```python
from build123d import *

# Parameters (mm, degrees)
F1_DEPTH     = 25.4
F2_R         = 17.018
F3_DEPTH     = 27.686
F4_R         = 35.7378
F5_DEPTH     = 24.638
F6_R         = 17.7830971004
F7_DEPTH     = 25.4
F8_W         = 71.4756
F8_H         = 155.2468025039
F9_DEPTH     = 24.638
F10_R        = 17.78
F12_T1_DEPTH = 35.9156
F12_T3_DEPTH = 26.5465599919
F12_T6_ANGLE = 90
F12_T8_ANGLE = 90


# Not quite as in the source:
# - a fillet or chamfer that OpenCascade refuses, or shapes differently, is made with other operations: its cross-section is extruded or revolved along the edge and cut away or added


with BuildPart() as f1:
    # F0 (on Top) → F1 (new body)
    with BuildSketch(Plane.XY):
        with BuildLine():
            Line((-43.18, 0), (43.18, 0))
            ThreePointArc((43.18, 0), (0, 43.18), (-43.18, 0))
        make_face()
        with BuildLine():
            ThreePointArc((-43.18, 0), (0, -43.18), (43.18, 0))
            Line((43.18, 0), (-43.18, 0))
        make_face()
    extrude(amount=F1_DEPTH)

    # F2 (on face) → F3 (cut)
    with BuildSketch(Plane.XY):
        Circle(F2_R)
    extrude(amount=F3_DEPTH, mode=Mode.SUBTRACT)

    # F4 (on face) → F5 (cut)
    with BuildSketch(Plane.XY.offset(25.4)):
        Circle(F4_R)
    extrude(amount=-F5_DEPTH, mode=Mode.SUBTRACT)

    # F6
    f6_edges = [f1.edges().sort_by_distance(p)[0] for p in [
        (-35.7378, 0, 0.762),
    ]]
    fillet(f6_edges, radius=F6_R)

    # F0 (on Top) → F7 (join)
    with BuildSketch(Plane.XY):
        with BuildLine():
            Line((43.18, -150.0849872828), (43.18, 0))
            ThreePointArc((43.18, 0), (0, -43.18), (-43.18, 0))
            Line((-43.18, 0), (-43.18, -150.0849872828))
            Line((-43.18, -150.0849872828), (43.18, -150.0849872828))
        make_face()
    extrude(amount=F7_DEPTH)

    # F8 (on face) → F9 (cut)
    with BuildSketch(Plane.XY.offset(25.4)):
        with Locations((0, -77.6234012519)):
            Rectangle(F8_W, F8_H)
    extrude(amount=-F9_DEPTH, mode=Mode.SUBTRACT)

    # F10
    f10_edges = [f1.edges().sort_by_distance(p)[0] for p in [
        (35.7378, -75.042494, 0.762),
        (-35.7378, -75.042494, 0.762),
    ]]
    fillet(f10_edges, radius=F10_R)

    # F11: chamfer of 5.08 on 1 edges, made by hand


with BuildPart() as f11_tool2:
    # F11_s3 → F11_t4 (revolve)
    with BuildSketch(Plane.XZ):
        with BuildLine():
            Line((23.1756307345, 1.8396307345), (15.9403692655, -5.3956307345))
            Line((15.9403692655, -5.3956307345), (15.1783692655, -5.3956307345))
            ThreePointArc((15.1783692655, -5.3956307345), (16.256, -2.3168153673), (16.256, 0.762))
            Line((16.256, 0.762), (17.018, 1.524))
            ThreePointArc((17.018, 1.524), (20.0968153673, 1.524), (23.1756307345, 2.6016307345))
            Line((23.1756307345, 2.6016307345), (23.1756307345, 1.8396307345))
        make_face()
    revolve(axis=Axis((0, 0, 0.762), (0, 0, -1)))

    split(bisect_by=Plane.XZ, keep=Keep.TOP)


with BuildPart() as f1_1:
    add(f1.part)

    # F11_t1: cut F11_tool2
    add(f11_tool2.part, mode=Mode.SUBTRACT)


with BuildPart() as f11_tool7:
    # F11_s8 → F11_t9 (revolve)
    with BuildSketch(Plane.XZ):
        with BuildLine():
            Line((23.1756307345, 1.8396307345), (15.9403692655, -5.3956307345))
            Line((15.9403692655, -5.3956307345), (15.1783692655, -5.3956307345))
            ThreePointArc((15.1783692655, -5.3956307345), (16.256, -2.3168153673), (16.256, 0.762))
            Line((16.256, 0.762), (17.018, 1.524))
            ThreePointArc((17.018, 1.524), (20.0968153673, 1.524), (23.1756307345, 2.6016307345))
            Line((23.1756307345, 2.6016307345), (23.1756307345, 1.8396307345))
        make_face()
    revolve(axis=Axis((0, 0, 0.762), (0, 0, -1)))

    split(bisect_by=Plane.XZ, keep=Keep.BOTTOM)


with BuildPart() as f1_2:
    add(f1_1.part)

    # F11_t6: cut F11_tool7
    add(f11_tool7.part, mode=Mode.SUBTRACT)

    # F12: chamfer of 5.08 x 7.62 on 5 edges, made by hand

    # F12_s2 → F12_t1 (cut)
    with BuildSketch(Plane.YZ.offset(-17.9578)):
        Polygon((-142.4649872828, 0.762), (-150.0849872828, -4.318), (-150.0849872828, 0.762), align=None)
    extrude(amount=F12_T1_DEPTH, mode=Mode.SUBTRACT)

    # F12_s4 → F12_t3 (cut)
    with BuildSketch(Plane.XY.offset(18.542)):
        Polygon((35.7378, -142.4649872828), (40.8178, -150.0849872828), (35.7378, -150.0849872828), align=None)
        Polygon((-35.7378, -142.4649872828), (-40.8178, -150.0849872828), (-35.7378, -150.0849872828), align=None)
    extrude(amount=F12_T3_DEPTH, mode=Mode.SUBTRACT)

    # F12_s5 → F12_t6 (revolve, cut)
    with BuildSketch(Plane.YZ.offset(-17.9578)):
        Polygon((-142.4649872828, 0.762), (-150.0849872828, -4.318), (-150.0849872828, 0.762), align=None)
    revolve(axis=Axis((-17.9578, -150.0849872828, 18.542), (0, 1, 0)), revolution_arc=F12_T6_ANGLE, mode=Mode.SUBTRACT)

    # F12_s7 → F12_t8 (revolve, cut)
    with BuildSketch(Plane.XY.offset(18.542)):
        Polygon((40.8178, -150.0849872828), (35.7378, -142.4649872828), (35.7378, -150.0849872828), align=None)
    revolve(axis=Axis((17.9578, -150.0849872828, 18.542), (0, 1, 0)), revolution_arc=F12_T8_ANGLE, mode=Mode.SUBTRACT)


solid = f1_2.part
```
Design review of the part built by this model. Coordinates are the model's own, in mm. A direction names the side the tool comes from. Coordinates: 2 decimals unless noted, no trailing zeros. Order: outer loops, then holes, each group sorted by start corner. A loop starts at its lowest first (then second) coordinate and runs counter-clockwise, first axis right, second up.
1) For faces 1 (the cylindrical face through (0.79, 35.73, 22.02)), 2 (the flat face through (-40, -150.085, 10)), list the 3-axis set-ups (+Z, -Z, +X, -X, +Y, -Y) from which the entire face can be reached by the end or side of a thin tool; tool diameter is ignored.
2) Take a section at A-A, the plane y = -38. Give the boundary of the cut face in (x, z).
3) Clearance check with flat-ended pins moving along their axes: pin 1 (1 mm diameter, centred on x = -23, z = 17, fed in from -Y); pin 2 (11 mm diameter, centred on x = 4, y = -85.5, fed in from +Z); pin 3 (10 mm diameter, centred on x = 6, z = 6, fed in from -Y); pin 4 (6 mm diameter, centred on x = 11, y = -11, fed in from -Z). State where each tip first meets the part, or that it passes through.
4) Wall thickness on line 1 along X through (y, z) = (-66.5, 17.75); line 2 along X through (y, z) = (-39.5, 7.5); line 3 along Z through (x, y) = (16.5, -52): over which ranges is each line inside the solid? List them lowest first.
5) Take a section at B-B, the plane x = 0. Give the boundary of the cut face in (y, z), and give its area (3 significant figures).
Returned:
1. face 1: +Z, -Y
1. face 2: +Z, -Z, +X, -X, -Y
2. outline: (-43.18, 0) - (43.18, 0) - (43.18, 25.4) - (35.74, 25.4) - (35.74, 18.54) arc R17.78 cw to (17.96, 0.76) - (-17.96, 0.76) arc R17.78 cw to (-35.74, 18.54) - (-35.74, 25.4) - (-43.18, 25.4) - close
3. pin 1: stops at y = 26.83
3. pin 2: stops at z = 0.76
3. pin 3: stops at y = 21.28
3. pin 4: passes through
4. line 1: x = -43.18 to -35.72, 35.72 to 43.18
4. line 2: x = -43.18 to -31.89, 31.89 to 43.18
4. line 3: z = 0 to 0.76
5. outline: (-143.61, 0) - (-21.34, 0) - (-22.1, 0.76) - (-142.46, 0.76) - close; (21.34, 0) - (43.18, 0) - (43.18, 25.4) - (35.74, 25.4) - (35.74, 18.55) arc R17.78 cw to (22.76, 1.42) - close
5. area: 359 mm2
